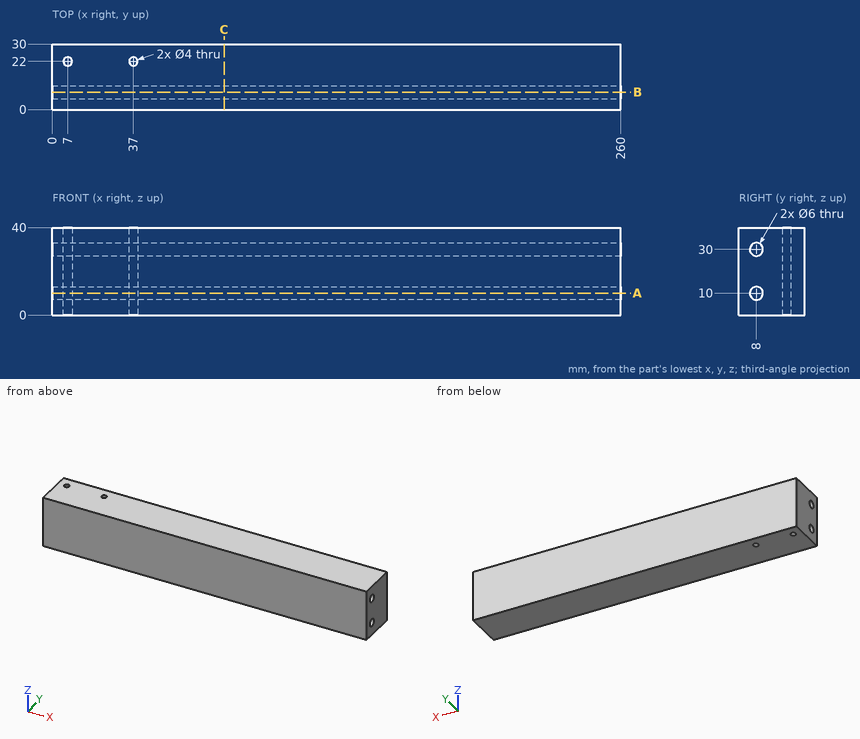
Check sheet for the drawn part. Datum: minimum x, y, z corner. Units: mm. Round coordinates to 2 decimals unless told otherwise and drop trailing zeros. Loops run counter-clockwise (first coordinate to the right, second up) from the corner with the lowest first, then second, coordinate; pieces in that order, holes last. Notation, with made-up numbers: (15.5, 87) - (36.5, 87) arc R6 cw to (36.5, 96) - close; hole circle Ø5 at (8.5, 20). An arc over 180 degrees is marked (long way). Write each question's results on one line, items separated by ' | '. Start each with the question number.
Q1. Cross-section at B-B on y = 8. Enter the section's corners in (x, z), and give its area (3 significant figures).
Q2. Gauge pin test, flat ends, axial feed: P1, Ø1, axis at y = 23, z = 19.5, coming from the -X side; P2, Ø3, axis at x = 37, y = 22, coming from the +Z side. Record the tip position at first contact, or that the pin passes through.
Q3. Thickness scan on line 1 (Y direction, x = 100.5, z = 30); line 2 (X direction, y = 23, z = 11); line 3 (Y direction, x = 35.5, z = 22). Record the ranges inside material, lowest first. Write a range as [from, to].
Q4. Cross-section at A-A on z = 10. Enter the section's corners in (x, y).
Q5. Cross-section at C-C on x = 78.5. Enter the section's corners in (y, z), and give its area (3 significant figures).
Answers below:
1) outline: (0, 0) - (260, 0) - (260, 7) - (0, 7) - close; (0, 13) - (260, 13) - (260, 27) - (0, 27) - close; (0, 33) - (260, 33) - (260, 40) - (0, 40) - close | area: 7,280 mm²
2) P1: stops at x = 0 | P2: passes through
3) line 1: y = [0, 5], [11, 30] | line 2: x = [0, 5.27], [8.73, 35.27], [38.73, 260] | line 3: y = [0, 20.68], [23.32, 30]
4) outline: (0, 0) - (260, 0) - (260, 5) - (0, 5) - close; (0, 11) - (260, 11) - (260, 30) - (0, 30) - close; hole circle Ø4 at (7, 22); hole circle Ø4 at (37, 22)
5) outline: (0, 0) - (30, 0) - (30, 40) - (0, 40) - close; hole circle Ø6 at (8, 10); hole circle Ø6 at (8, 30) | area: 1,140 mm²
